Job drawing, mm, ordinate dimensions from the low corner. One solid piece. Coordinates: 2 decimals unless noted, no trailing zeros. Order: outer loops, then holes, each group sorted by start corner. A loop starts at its lowest first (then second) coordinate and runs counter-clockwise, first axis right, second up. Notation, with made-up numbers: (82, -23) - (120, -23) arc R35 cw to (120, 13) - close; hole circle Ø3 at (84, 4.5). An arc over 180 degrees is marked (long way). Use one line per item in the form item = value.
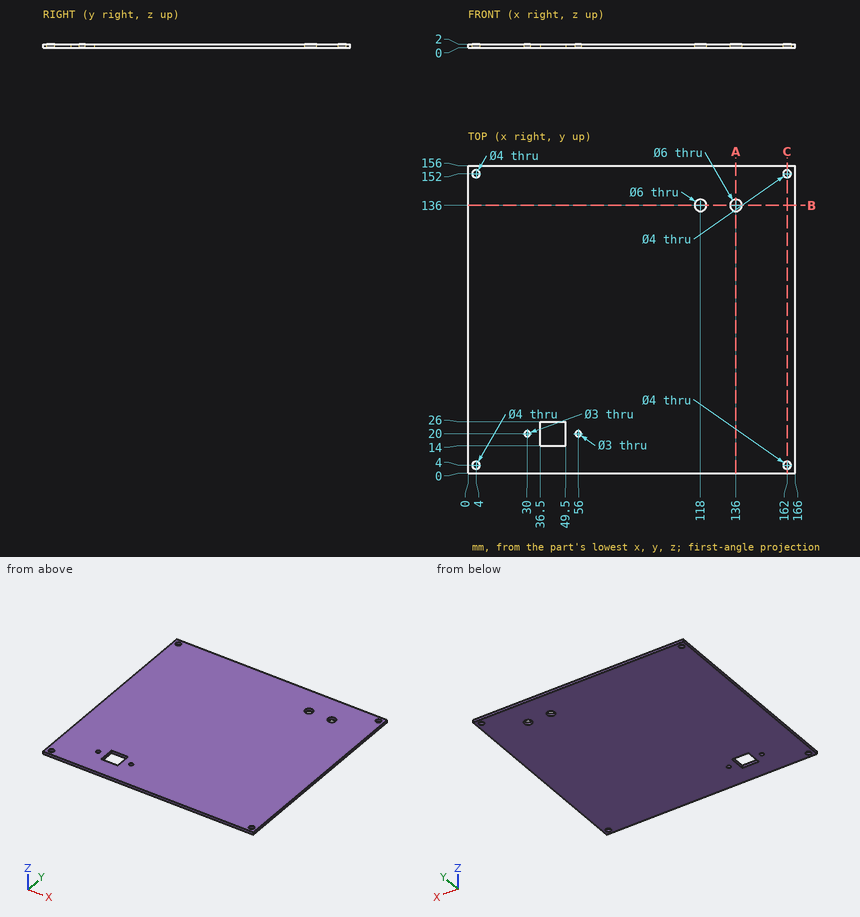
Item 1: Cut at B-B, the plane y = 136. Write the cut outline in (x, z).
Derived:
outline = (0, 0) - (115, 0) - (115, 2) - (0, 2) - close; (121, 0) - (133, 0) - (133, 2) - (121, 2) - close; (139, 0) - (166, 0) - (166, 2) - (139, 2) - close
Item 2: Cut at A-A, the plane x = 136. Write the cut outline in (y, z), plus the area to 3 significant figures.
Derived:
outline = (0, 0) - (133, 0) - (133, 2) - (0, 2) - close; (139, 0) - (156, 0) - (156, 2) - (139, 2) - close
area = 300 mm²
Item 3: Drill centre lines: line 1 (X direction, y = 136, z = 0.9); line 2 (Y direction, x = 162, z = 1.2); line 3 (X direction, y = 152, z = 1.4). Where is each one in solid material? Low to high. Write a range as [from, to].
Derived:
line_1 = [0, 115], [121, 133], [139, 166]
line_2 = [0, 2], [6, 150], [154, 156]
line_3 = [0, 2], [6, 160], [164, 166]
Item 4: Cut at C-C, the plane x = 162. Write the cut outline in (y, z), plus the area to 3 significant figures.
Derived:
outline = (0, 0) - (2, 0) - (2, 2) - (0, 2) - close; (6, 0) - (150, 0) - (150, 2) - (6, 2) - close; (154, 0) - (156, 0) - (156, 2) - (154, 2) - close
area = 296 mm²
